For this review, take the finished solid that the model builds, in its own axes (mm). A direction names the side the tool comes from. Give positions to 0.01 mm unless a question says otherwise; leave off trailing zeros. Loops run counter-clockwise (first coordinate to the right, second up) from the corner with the lowest first, then second, coordinate; pieces in that order, holes last. Notation, with made-up numbers: M 29,23.5 L 73,23.5 A31 cw 73,55.5 Z; hole C 37.5,-30.5 d7. An arc over 180 degrees is marked long. Use CSV: the item, a comma, the result in double quotes. Start each with the question number.
1. Take a section at B-B, the plane x = 0. Write out the cut boundary in (y, z), and give its area (3 significant figures).
2. Take a section at C-C, the plane z = 0. Write out the cut boundary in (x, y).
3. Take a section at A-A, the plane z = -10.5. Write out the cut boundary in (x, y).
4. Tool access review of faces 4 (the face through (0.83, 13.31, -11.13)), 5 (the face through (-6, 30, 0)), 6 (the face through (11.17, 13.311, -0.816)): name each direction out of +Z, -Z, +X, -X, +Y, -Y from which nothing blocks a thin tool from reaching the whole face with its end or side.
5. Insertion check: P1, Ø1, axis at x = 7.5, y = 10.5, coming from the +Z side; P2, Ø1.5, axis at x = 7.5, y = 16, coming from the +Z side; P3, Ø5, axis at x = -1, z = -10, coming from the +Y side. Each pin has a flat end and moves straight along its axis. Give the tip position at first contact, or say it passes through.
6. To check wall thickness, follow line 1 (Z direction, x = -9, y = 6); line 2 (Z direction, x = 0.25, y = 29.5); line 3 (Y direction, x = -7.75, z = -6.5). State the ranges of each line that lie inside material, in increasing order. Write a range as [from, to].
7. The part is to be moulded in two halves that separate along Z. For faces 1 (the face through (-2, 13.3, 9.8)), 2 (the face through (-1.94, 13.31, -9.81)), 3 (the face through (-10.63, 13.31, -3.52)), say which applies: pulls with the +Z half, pulls with the -Z half, needs draft (parallel to the pull), parting line crosses it, or undercut.
8. Take a section at D-D, the plane y = 28.5. Write out the cut boundary in (x, z), and give its area (3 significant figures).
from build123d import *

# Parameters (mm, degrees)
BOSS_EXTRUDE1_DEPTH = 27
SKETCH2_R           = 6
BOSS_EXTRUDE2_DEPTH = 4
SKETCH4_R           = 7
BOSS_EXTRUDE3_DEPTH = 1
SKETCH5_R           = 6
BOSS_EXTRUDE4_DEPTH = 1
CHAMFER1_SIZE       = 0.5


with BuildPart() as part:
    # Sketch1 → Boss-Extrude1 (new body)
    with BuildSketch(Plane(origin=(0, 0, 0), x_dir=(1, 0, 0), z_dir=(0, 1, 0))):
        with BuildLine():
            Line((0.5, 12.489995997), (-0.5, 12.489995997))
            ThreePointArc((-0.5, 12.489995997), (-0.822089844, 11.151281888), (-1.4, 9.901515036))
            ThreePointArc((-1.4, 9.901515036), (-1.95090322, 9.807852804), (-2.495714414, 9.683563888))
            ThreePointArc((-2.495714414, 9.683563888), (-3.507898848, 10.61704126), (-4.317774772, 11.730593379))
            Line((-4.317774772, 11.730593379), (-5.241654305, 11.347909946))
            ThreePointArc((-5.241654305, 11.347909946), (-5.026922808, 9.987840934), (-5.082577105, 8.612050277))
            ThreePointArc((-5.082577105, 8.612050277), (-5.55570233, 8.314696123), (-6.011478932, 7.991377919))
            ThreePointArc((-6.011478932, 7.991377919), (-7.303841738, 8.466452345), (-8.478207476, 9.185314257))
            Line((-8.478207476, 9.185314257), (-9.185314257, 8.478207476))
            ThreePointArc((-9.185314257, 8.478207476), (-8.466452345, 7.303841738), (-7.991377919, 6.011478932))
            ThreePointArc((-7.991377919, 6.011478932), (-8.314696123, 5.55570233), (-8.612050277, 5.082577105))
            ThreePointArc((-8.612050277, 5.082577105), (-9.987840934, 5.026922808), (-11.347909946, 5.241654305))
            Line((-11.347909946, 5.241654305), (-11.730593379, 4.317774772))
            ThreePointArc((-11.730593379, 4.317774772), (-10.61704126, 3.507898848), (-9.683563888, 2.495714414))
            ThreePointArc((-9.683563888, 2.495714414), (-9.807852804, 1.95090322), (-9.901515036, 1.4))
            ThreePointArc((-9.901515036, 1.4), (-11.151281888, 0.822089844), (-12.489995997, 0.5))
            Line((-12.489995997, 0.5), (-12.489995997, -0.5))
            ThreePointArc((-12.489995997, -0.5), (-11.151281888, -0.822089844), (-9.901515036, -1.4))
            ThreePointArc((-9.901515036, -1.4), (-9.807852804, -1.95090322), (-9.683563888, -2.495714414))
            ThreePointArc((-9.683563888, -2.495714414), (-10.61704126, -3.507898848), (-11.730593379, -4.317774772))
            Line((-11.730593379, -4.317774772), (-11.347909946, -5.241654305))
            ThreePointArc((-11.347909946, -5.241654305), (-9.987840934, -5.026922808), (-8.612050277, -5.082577105))
            ThreePointArc((-8.612050277, -5.082577105), (-8.314696123, -5.55570233), (-7.991377919, -6.011478932))
            ThreePointArc((-7.991377919, -6.011478932), (-8.466452345, -7.303841738), (-9.185314257, -8.478207476))
            Line((-9.185314257, -8.478207476), (-8.478207476, -9.185314257))
            ThreePointArc((-8.478207476, -9.185314257), (-7.303841738, -8.466452345), (-6.011478932, -7.991377919))
            ThreePointArc((-6.011478932, -7.991377919), (-5.55570233, -8.314696123), (-5.082577105, -8.612050277))
            ThreePointArc((-5.082577105, -8.612050277), (-5.026922808, -9.987840934), (-5.241654305, -11.347909946))
            Line((-5.241654305, -11.347909946), (-4.317774772, -11.730593379))
            ThreePointArc((-4.317774772, -11.730593379), (-3.507898848, -10.61704126), (-2.495714414, -9.683563888))
            ThreePointArc((-2.495714414, -9.683563888), (-1.95090322, -9.807852804), (-1.4, -9.901515036))
            ThreePointArc((-1.4, -9.901515036), (-0.822089844, -11.151281888), (-0.5, -12.489995997))
            Line((-0.5, -12.489995997), (0.5, -12.489995997))
            ThreePointArc((0.5, -12.489995997), (0.822089844, -11.151281888), (1.4, -9.901515036))
            ThreePointArc((1.4, -9.901515036), (1.95090322, -9.807852804), (2.495714414, -9.683563888))
            ThreePointArc((2.495714414, -9.683563888), (3.507898848, -10.61704126), (4.317774772, -11.730593379))
            Line((4.317774772, -11.730593379), (5.241654305, -11.347909946))
            ThreePointArc((5.241654305, -11.347909946), (5.026922808, -9.987840934), (5.082577105, -8.612050277))
            ThreePointArc((5.082577105, -8.612050277), (5.55570233, -8.314696123), (6.011478932, -7.991377919))
            ThreePointArc((6.011478932, -7.991377919), (7.303841738, -8.466452345), (8.478207476, -9.185314257))
            Line((8.478207476, -9.185314257), (9.185314257, -8.478207476))
            ThreePointArc((9.185314257, -8.478207476), (8.466452345, -7.303841738), (7.991377919, -6.011478932))
            ThreePointArc((7.991377919, -6.011478932), (8.314696123, -5.55570233), (8.612050277, -5.082577105))
            ThreePointArc((8.612050277, -5.082577105), (9.987840934, -5.026922808), (11.347909946, -5.241654305))
            Line((11.347909946, -5.241654305), (11.730593379, -4.317774772))
            ThreePointArc((11.730593379, -4.317774772), (10.61704126, -3.507898848), (9.683563888, -2.495714414))
            ThreePointArc((9.683563888, -2.495714414), (9.807852804, -1.95090322), (9.901515036, -1.4))
            ThreePointArc((9.901515036, -1.4), (11.151281888, -0.822089844), (12.489995997, -0.5))
            Line((12.489995997, -0.5), (12.489995997, 0.5))
            ThreePointArc((12.489995997, 0.5), (11.151281888, 0.822089844), (9.901515036, 1.4))
            ThreePointArc((9.901515036, 1.4), (9.807852804, 1.95090322), (9.683563888, 2.495714414))
            ThreePointArc((9.683563888, 2.495714414), (10.61704126, 3.507898848), (11.730593379, 4.317774772))
            Line((11.730593379, 4.317774772), (11.347909946, 5.241654305))
            ThreePointArc((11.347909946, 5.241654305), (9.987840934, 5.026922808), (8.612050277, 5.082577105))
            ThreePointArc((8.612050277, 5.082577105), (8.314696123, 5.55570233), (7.991377919, 6.011478932))
            ThreePointArc((7.991377919, 6.011478932), (8.466452345, 7.303841738), (9.185314257, 8.478207476))
            Line((9.185314257, 8.478207476), (8.478207476, 9.185314257))
            ThreePointArc((8.478207476, 9.185314257), (7.303841738, 8.466452345), (6.011478932, 7.991377919))
            ThreePointArc((6.011478932, 7.991377919), (5.55570233, 8.314696123), (5.082577105, 8.612050277))
            ThreePointArc((5.082577105, 8.612050277), (5.026922808, 9.987840934), (5.241654305, 11.347909946))
            Line((5.241654305, 11.347909946), (4.317774772, 11.730593379))
            ThreePointArc((4.317774772, 11.730593379), (3.507898848, 10.61704126), (2.495714414, 9.683563888))
            ThreePointArc((2.495714414, 9.683563888), (1.95090322, 9.807852804), (1.4, 9.901515036))
            ThreePointArc((1.4, 9.901515036), (0.822089844, 11.151281888), (0.5, 12.489995997))
        make_face()
    extrude(amount=BOSS_EXTRUDE1_DEPTH)

    # Sketch2 → Boss-Extrude2 (add)
    with BuildSketch(Plane(origin=(0, 27, 0), x_dir=(1, 0, 0), z_dir=(0, 1, 0))):
        Circle(SKETCH2_R)
    extrude(amount=BOSS_EXTRUDE2_DEPTH)

    # Sketch4 → Boss-Extrude3 (add)
    with BuildSketch(Plane(origin=(0, 27, 0), x_dir=(1, 0, 0), z_dir=(0, 1, 0))):
        Circle(SKETCH4_R)
    extrude(amount=BOSS_EXTRUDE3_DEPTH)

    # Sketch5 → Boss-Extrude4 (add)
    with BuildSketch(Plane(origin=(0, 31, 0), x_dir=(1, 0, 0), z_dir=(0, 1, 0))):
        Circle(SKETCH5_R)
    extrude(amount=BOSS_EXTRUDE4_DEPTH)

    # Chamfer1
    chamfer1_edges = [part.edges().sort_by_distance(p)[0] for p in [
        (-7, 28, 0),
    ]]
    chamfer(chamfer1_edges, length=CHAMFER1_SIZE)


solid = part.part
Result set:
1,outline,"M 0,-12.49 L 27,-12.49 L 27,-7 L 27.5,-7 L 28,-6.5 L 28,-6 L 32,-6 L 32,6 L 28,6 L 28,6.5 L 27.5,7 L 27,7 L 27,12.49 L 0,12.49 Z"
1,area,"736 mm2"
2,outline,"M -12.49,0 L 12.49,0 L 12.49,27 L 7,27 L 7,27.5 L 6.5,28 L 6,28 L 6,32 L -6,32 L -6,28 L -6.5,28 L -7,27.5 L -7,27 L -12.49,27 Z"
3,outline,"M -5.08,0 L -3.4,0 L -3.4,27 L -5.08,27 Z; M -1.09,0 L 1.09,0 L 1.09,27 L -1.09,27 Z; M 3.4,0 L 5.08,0 L 5.08,27 L 3.4,27 Z"
4,face 4,"-Z, +Y, -Y"
4,face 5,"+Y"
4,face 6,"+X, +Y, -Y"
5,P1,"z = 8.85"
5,P2,"z = 9.02"
5,P3,"y = 27"
6,line 1,"[-8.66, -8.22], [-5.04, 5.04], [8.22, 8.66]"
6,line 2,"[-5.99, 5.99]"
6,line 3,"[0, 27]"
7,face 1,"pulls with the +Z half"
7,face 2,"pulls with the -Z half"
7,face 3,"undercut"
8,outline,"C 0,0 d12"
8,area,"113 mm2"
